```python
from build123d import *
from build123d.topology import SkipClean

# Parameters (mm, degrees)
SKETCH13_R                                  = 3
HEAD_PIN_DEPTH                              = 5
SKETCH2_W                                   = 6
SKETCH2_H                                   = 6
HIP_HOLE_PART_1_DEPTH                       = 2.5
SKETCH3_W                                   = 6
SKETCH3_H                                   = 6
HIP_HOLE_PART_2_DEPTH                       = 2.5
HIP_HOLE_PART_2_DRAFT                       = -10
SKETCH14_R                                  = 1.9
ARM_PIN_DEPTH                               = 4.5
ARM_START                                   = -1
ARM_POSITION_SLOT_DEPTH                     = 1
EASY_ARM_INSERT_R                           = 0.5
COPYING_OVER_ARM_AND_HIP_CONNECTORS_COPY_W  = 6
COPYING_OVER_ARM_AND_HIP_CONNECTORS_COPY_H  = 6
COPYING_OVER_ARM_AND_HIP_CONNECTORS_2_DEPTH = 2.5
COPYING_OVER_ARM_AND_HIP_CONNECTORS_2_DRAFT = -10
EASY_ARM_INSERT_OF_COPYING_OVER_ARM_AND_R   = 0.5
EASY_HEAD_INSERT_R                          = 0.5
SCALE1_SCALE                                = 2


with BuildPart() as part:
    # 3DSketch1 → Body section 0
    with BuildSketch(Plane(origin=(10, 20, -1.25), x_dir=(-0.9363291775690445, 0, -0.35112344158839165), z_dir=(0, -1, 0))):
        with BuildLine():
            Line((0, 0), (2.633425812, 7.022468832))
            Line((2.633425812, 7.022468832), (21.360009363, 0))
            Line((21.360009363, 0), (18.726583551, -7.022468832))
            Line((18.726583551, -7.022468832), (0, 0))
        make_face()
    # Sketch1 → Body section 1
    with BuildSketch(Plane(origin=(0, 0, 0), x_dir=(1, 0, 0), z_dir=(0, 1, 0))):
        with BuildLine():
            Line((-10, 0), (10, 0))
            Line((10, 0), (10, 10))
            Line((10, 10), (-10, 10))
            Line((-10, 10), (-10, 0))
        make_face()
    loft()

    # Sketch13 → Head pin (add)
    with BuildSketch(Plane(origin=(0, 20, 0), x_dir=(1, 0, 0), z_dir=(0, 1, 0))):
        with Locations(Location((0, 5, 0), (0, 0, 270))):
            Circle(SKETCH13_R)
    extrude(amount=HEAD_PIN_DEPTH)

    # Sketch2 → Hip hole part 1 (cut)
    with BuildSketch(Plane(origin=(0, 0, 0), x_dir=(-1, 0, 0), z_dir=(0, -1, 0))):
        with Locations((-5, 5)):
            Rectangle(SKETCH2_W, SKETCH2_H)
    hip_hole_part_1 = extrude(amount=-HIP_HOLE_PART_1_DEPTH, mode=Mode.SUBTRACT)


with BuildPart() as hip_hole_part_2_tool:
    # Sketch3 → Hip hole part 2 (with draft: the straight prism first)
    with BuildSketch(Plane.XZ.offset(-2.5)):
        with Locations((5, -5)):
            Rectangle(SKETCH3_W, SKETCH3_H)
    extrude(amount=-HIP_HOLE_PART_2_DEPTH)
    # Hip hole part 2: the draft: its side faces are tilted about the plane it starts from
    hip_hole_part_2_sides = [hip_hole_part_2_tool.faces().sort_by_distance(p)[0] for p in [
        (8, 3.75, -5),
        (5, 3.75, -2),
        (2, 3.75, -5),
        (5, 3.75, -8),
    ]]
    draft(hip_hole_part_2_sides, Plane.XZ.offset(-2.5), HIP_HOLE_PART_2_DRAFT)


with BuildPart() as part_1:
    add(part.part)

    # Hip hole part 2: cut by hip_hole_part_2_tool
    add(hip_hole_part_2_tool.part, mode=Mode.SUBTRACT)

    # Sketch18 → Weight reduction/Make it easy to add centerlines (revolve, cut)
    with BuildSketch(Plane(origin=(5, 5, -5), x_dir=(0, 0, -1), z_dir=(1, 0, 0))):
        Polygon((0, 0), (0, 2.901290929), (1.5, 2), (1.5, 0), align=None)
    weight_reduction_make_it_easy_to_add_cen = revolve(axis=Axis((5, -1.35, -5), (0, 1, 0)), mode=Mode.SUBTRACT)

    # Sketch14 → Arm pin (add)
    with BuildSketch(Plane(origin=(10, 0, 0), x_dir=(0, 0, -1), z_dir=(1, 0, 0))):
        with Locations(Location((5, 16.75, 0), (0, 0, 90))):
            Circle(SKETCH14_R)
    arm_pin = extrude(amount=ARM_PIN_DEPTH)

    # Sketch15 → Arm position slot (cut)
    with SkipClean():  # the faces are left unmerged after this step: merging them gives an invalid solid
        with BuildSketch(Plane(origin=(10, 0, 0), x_dir=(0, 0, -1), z_dir=(1, 0, 0)).offset(ARM_START)):
            with BuildLine():
                ThreePointArc((2.807968978, 18.942031022), (3.689883389, 13.94044586), (8.088203564, 16.479817197))
                ThreePointArc((8.088203564, 16.479817197), (7.542780191, 17.129827462), (6.892769926, 16.584404089))
                ThreePointArc((6.892769926, 16.584404089), (4.197025303, 15.028015205), (3.656497116, 18.093502884))
                ThreePointArc((3.656497116, 18.093502884), (3.656497116, 18.942031022), (2.807968978, 18.942031022))
            make_face()
        arm_position_slot = extrude(amount=ARM_POSITION_SLOT_DEPTH, mode=Mode.SUBTRACT)

    # Easy arm insert
    easy_arm_insert_edges = [part_1.edges().sort_by_distance(p)[0] for p in [
        (14.5, 14.85, -5),
    ]]
    fillet(easy_arm_insert_edges, radius=EASY_ARM_INSERT_R)

    # Copying over arm and hip connectors: Hip hole part 1, Weight reduction/Make it easy to add centerlines, Arm pin, Arm position slot across plane
    with SkipClean():  # the faces are left unmerged after this step: merging them gives an invalid solid
        add(hip_hole_part_1.mirror(Plane(origin=(0, 0, 0), x_dir=(0, 0, 1), z_dir=(1, 0, 0))), mode=Mode.SUBTRACT)
        add(weight_reduction_make_it_easy_to_add_cen.mirror(Plane(origin=(0, 0, 0), x_dir=(0, 0, 1), z_dir=(1, 0, 0))), mode=Mode.SUBTRACT)
        add(arm_pin.mirror(Plane(origin=(0, 0, 0), x_dir=(0, 0, 1), z_dir=(1, 0, 0))))
        add(arm_position_slot.mirror(Plane(origin=(0, 0, 0), x_dir=(0, 0, 1), z_dir=(1, 0, 0))), mode=Mode.SUBTRACT)


with BuildPart() as copying_over_arm_and_hip_connectors_2_tool:
    # Copying over arm and hip connectors copy → Copying over arm and hip connectors  2 (with draft: the straight prism first)
    with BuildSketch(Plane(origin=(0, 2.5, 0), x_dir=(-1, 0, 0), z_dir=(0, -1, 0))):
        with Locations((5, 5)):
            Rectangle(COPYING_OVER_ARM_AND_HIP_CONNECTORS_COPY_W, COPYING_OVER_ARM_AND_HIP_CONNECTORS_COPY_H)
    extrude(amount=-COPYING_OVER_ARM_AND_HIP_CONNECTORS_2_DEPTH)
    # Copying over arm and hip connectors  2: the draft: its side faces are tilted about the plane it starts from
    copying_over_arm_and_hip_connectors_2_sides = [copying_over_arm_and_hip_connectors_2_tool.faces().sort_by_distance(p)[0] for p in [
        (-8, 3.75, -5),
        (-5, 3.75, -2),
        (-2, 3.75, -5),
        (-5, 3.75, -8),
    ]]
    draft(copying_over_arm_and_hip_connectors_2_sides, Plane(origin=(0, 2.5, 0), x_dir=(-1, 0, 0), z_dir=(0, -1, 0)), COPYING_OVER_ARM_AND_HIP_CONNECTORS_2_DRAFT)


with BuildPart() as part_2:
    add(part_1.part)

    # Copying over arm and hip connectors  2: cut by copying_over_arm_and_hip_connectors_2_tool
    add(copying_over_arm_and_hip_connectors_2_tool.part, mode=Mode.SUBTRACT)

    # Easy arm insert of Copying over arm and
    easy_arm_insert_of_copying_over_arm_and_edges = [part_2.edges().sort_by_distance(p)[0] for p in [
        (-14.5, 14.85, -5),
    ]]
    fillet(easy_arm_insert_of_copying_over_arm_and_edges, radius=EASY_ARM_INSERT_OF_COPYING_OVER_ARM_AND_R)

    # Easy head insert
    easy_head_insert_edges = [part_2.edges().sort_by_distance(p)[0] for p in [
        (0, 25, -8),
    ]]
    fillet(easy_head_insert_edges, radius=EASY_HEAD_INSERT_R)


with BuildPart() as part_3:
    # Scale1: scaled about (2e-09, 10.984808506, -5.003313796)
    add(part_2.part.scale(SCALE1_SCALE).moved(Location((-2e-09, -10.984808506, 5.003313796))))


solid = part_3.part
```
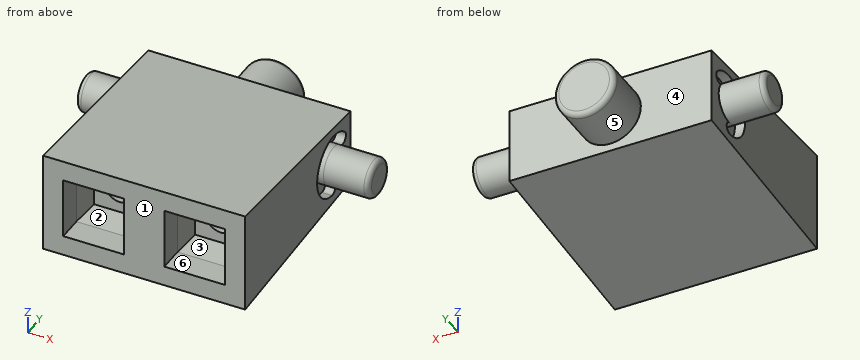
For this review, take the finished solid that the model builds, in its own axes (mm). Face numbers are marked on the shaded views. A direction names the side the tool comes from. Round coordinates to 2 decimals unless told otherwise and drop trailing zeros. Write each loop counter-clockwise with the first axis right and the second up, starting at its lowest first coordinate (ties: lowest second). Pieces come first, ordered by that corner, then holes. Notation, with made-up numbers: (16, 0) - (27, 0) arc R23 cw to (27, 28) - close; hole circle Ø9 at (-30.5, 82). An arc over 180 degrees is marked (long way). Answer as CSV lines item,"result". Start each with the question number.
(1) Machinability: for the marked faces 1 and 2, which of the approach directions +Z, -Z, +X, -X, +Y, -Y give a long, thin tool a straight path to every point of the face, cutting with its end or side? Answer none if there is none.
(2) Add section A-A, the plane x = 22. State the section outline as (y, z) points.
(3) For pin 1 (2 mm diameter, centred on x = 8.5, y = 27.5, fed in from +Z); pin 2 (1.5 mm diameter, centred on y = -9, z = -6, fed in from -X); pin 3 (1 mm diameter, centred on x = 21, z = -6.5, fed in from -Y); pin 4 (5.5 mm diameter, centred on x = -9.5, y = -9.5, fed in from -Z), all flat-tipped, find the tip position at first contact; note any pin that passes through.
(4) For line 1 (Y direction, x = -5, z = -0.75); line 2 (Y direction, x = -1.5, z = -12); line 3 (X direction, y = -1.5, z = -11.25), list the stretches that pass through material, from the lowest coordinate up.
(5) Mouldability with a two-part tool opening along X and no side actions: class the marked faces 3, 4, 5 and 6 as +X half, -X half, draft (parallel to the pull), parting line (faces both ways), or undercut.
From the geometry:
1,face 1,"+Z, -Z, +X, -X, -Y"
1,face 2,"-Y"
2,outline,"circle Ø7.6 at (22.52, -5)"
3,pin 1,"stops at z = 2.66"
3,pin 2,"stops at x = -20"
3,pin 3,"stops at y = 18.85"
3,pin 4,"stops at z = -15"
4,line 1,"y = -0.98 to 29.02"
4,line 2,"y = -10.98 to 29.02"
4,line 3,"x = -20 to 20"
5,face 3,"undercut"
5,face 4,"draft"
5,face 5,"parting line"
5,face 6,"undercut"
